Read the model definition and answer for the solid it produces. Units are mm, in the model's axes. Face numbers are marked on the shaded views. A direction names the side the tool comes from. Give positions to 0.01 mm unless a question says otherwise; leave off trailing zeros. Order: outer loops, then holes, each group sorted by start corner. A loop starts at its lowest first (then second) coordinate and runs counter-clockwise, first axis right, second up. Notation, with made-up numbers: (-16, 60.25) -> (42, 60.25) arc R27 cw to (42, 86.25) -> close; hole circle Ø3 at (4, 61). An arc over 180 degrees is marked (long way). Answer as CSV lines item,"result". Start each with the question number.
1) Find section D-D (z = 10.5). Determine the outline of the cut face in (x, y) (3 decimals).
2) Find section C-C (y = 7). Determine the outline of the cut face in (x, z).
3) Find section A-A (x = 0). Determine the outline of the cut face in (y, z) (3 decimals).
4) Flat-ended cylindrical pins translate along their axes: pin 1 Ø1.8 at (x, z) = (0, 56.5) entering from -Y (3 decimals); pin 2 Ø6.5 at (x, z) = (-0.5, 66) entering from +Y (3 decimals); pin 3 Ø2 at (x, z) = (-4, 50.5) entering from -Y. Find the tip coordinate at first contact, or state that the pin passes through.
5) Straight lines are drawn through the part: L1, parallel to Z at x = 8.75, y = 3; L2, parallel to Y at x = 1.25, z = 66.5 (3 decimals); L3, parallel to Y at x = 0.25, z = 26. For each, find the intervals that lie inside material, in ascending order. Write a range as from..to.
6) Find section B-B (z = 62.5). Determine the outline of the cut face in (x, y) (3 decimals), and give its area (3 significant figures).
7) For the marked faces 1, 2 and 3, determine the directions among +Z, -Z, +X, -X, +Y, -Y from which every point of the face is accessible in a straight line to the end or side of a thin tool.
```python
from build123d import *

# Parameters (mm, degrees)
F0_R     = 9.525
F1_DEPTH = 50.8
F3_DEPTH = 10
F5_DEPTH = 10
F6_SIZE  = 0.25


with BuildPart() as f1:
    # F0 (on Top) → F1 (new body)
    with BuildSketch(Plane.XY):
        Circle(F0_R)
    extrude(amount=F1_DEPTH)

    # F2 (on face) → F3 (join)
    with BuildSketch(Plane.XY.offset(50.8)):
        with BuildLine():
            Line((0, 6.025), (0, 0))
            Line((0, 0), (3, 0))
            Line((3, 0), (9.025, 0))
            ThreePointArc((9.025, 0), (7.260318, 4.260318), (3, 6.025))
            Line((3, 6.025), (0, 6.025))
        make_face()
        with BuildLine():
            Line((0, -6.025), (0, 0))
            Line((0, 0), (-3, 0))
            Line((-3, 0), (-9.025, 0))
            ThreePointArc((-9.025, 0), (-7.260318, -4.260318), (-3, -6.025))
            Line((-3, -6.025), (0, -6.025))
        make_face()
        with BuildLine():
            Line((-3, 0), (0, 0))
            Line((0, 0), (0, 6.025))
            Line((0, 6.025), (-3, 6.025))
            ThreePointArc((-3, 6.025), (-7.260318, 4.260318), (-9.025, 0))
            Line((-9.025, 0), (-3, 0))
        make_face()
        with BuildLine():
            Line((3, 0), (0, 0))
            Line((0, 0), (0, -6.025))
            Line((0, -6.025), (3, -6.025))
            ThreePointArc((3, -6.025), (7.260318, -4.260318), (9.025, 0))
            Line((9.025, 0), (3, 0))
        make_face()
    extrude(amount=F3_DEPTH)

    # F4 (on face) → F5 (join)
    with BuildSketch(Plane.XY.offset(60.8)):
        with BuildLine():
            Line((0, 5.975), (0, 0))
            Line((0, 0), (3, 0))
            Line((3, 0), (8.975, 0))
            ThreePointArc((8.975, 0), (7.224963, 4.224963), (3, 5.975))
            Line((3, 5.975), (0, 5.975))
        make_face()
        with BuildLine():
            Line((0, -5.975), (0, 0))
            Line((0, 0), (-3, 0))
            Line((-3, 0), (-8.975, 0))
            ThreePointArc((-8.975, 0), (-7.224963, -4.224963), (-3, -5.975))
            Line((-3, -5.975), (0, -5.975))
        make_face()
        with BuildLine():
            Line((-3, 0), (0, 0))
            Line((0, 0), (0, 5.975))
            Line((0, 5.975), (-3, 5.975))
            ThreePointArc((-3, 5.975), (-7.224963, 4.224963), (-8.975, 0))
            Line((-8.975, 0), (-3, 0))
        make_face()
        with BuildLine():
            Line((3, 0), (0, 0))
            Line((0, 0), (0, -5.975))
            Line((0, -5.975), (3, -5.975))
            ThreePointArc((3, -5.975), (7.224963, -4.224963), (8.975, 0))
            Line((8.975, 0), (3, 0))
        make_face()
    extrude(amount=F5_DEPTH)

    # F6
    f6_edges = [f1.edges().sort_by_distance(p)[0] for p in [
        (0, -5.975, 70.8),
    ]]
    chamfer(f6_edges, length=F6_SIZE)


solid = f1.part
```
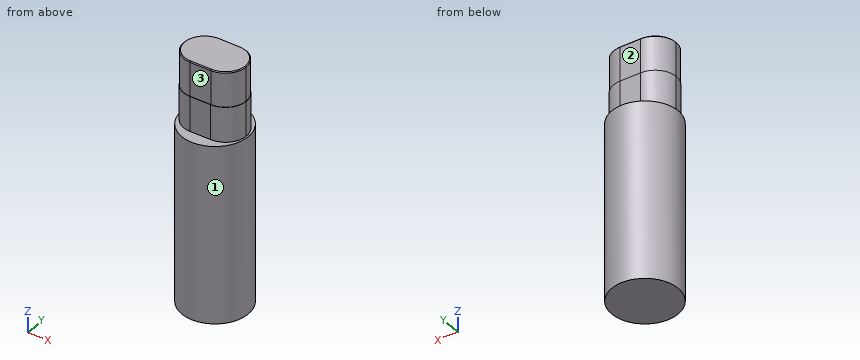
Findings below:
1,outline,"circle Ø19.05 at (0, 0)"
2,outline,"(-6.46, 0) -> (6.46, 0) -> (6.46, 50.8) -> (-6.46, 50.8) -> close"
3,outline,"(-9.525, 0) -> (9.525, 0) -> (9.525, 50.8) -> (6.025, 50.8) -> (6.025, 60.8) -> (5.975, 60.8) -> (5.975, 70.55) -> (5.725, 70.8) -> (-5.725, 70.8) -> (-5.975, 70.55) -> (-5.975, 60.8) -> (-6.025, 60.8) -> (-6.025, 50.8) -> (-9.525, 50.8) -> close"
4,pin 1,"y = -6.025"
4,pin 2,"y = 5.975"
4,pin 3,"y = -9.04"
5,L1,"0..50.8"
5,L2,"-5.975..5.975"
5,L3,"-9.52..9.52"
6,outline,"(-3, -5.975) -> (3, -5.975) arc R5.975 ccw to (3, 5.975) -> (-3, 5.975) arc R5.975 ccw to start"
6,area,"184 mm²"
7,face 1,"+Z, -Z"
7,face 2,"+Z, +X, -X, +Y"
7,face 3,"+Z, +X, -X, -Y"
